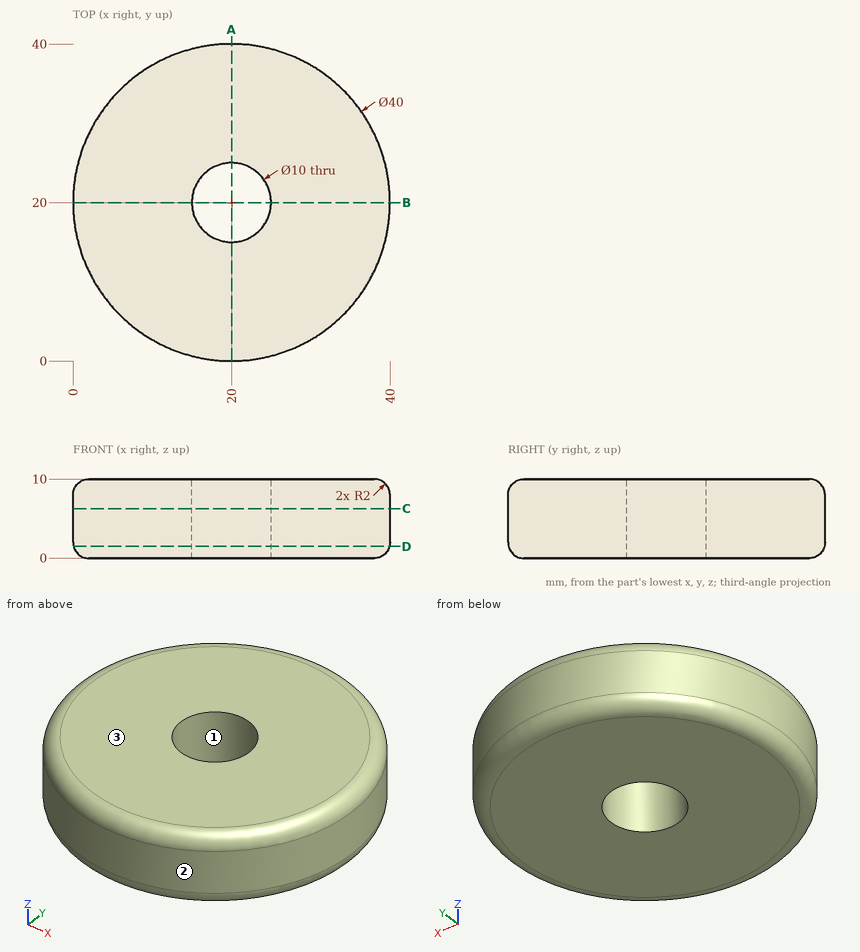
Geometry: see drawing. Coordinates: mm, zero at the bounding-box minimum. Round coordinates to 2 decimals unless told otherwise and drop trailing zeros. Loops run counter-clockwise (first coordinate to the right, second up) from the corner with the lowest first, then second, coordinate; pieces in that order, holes last. Notation, with made-up numbers: (38.5, 11.5) - (50.5, 11.5) arc R18 cw to (50.5, 32.5) - close; hole circle Ø5 at (29.25, -25). An arc over 180 degrees is marked (long way). Use CSV: the item, a comma, the result in double quotes.
Q1. Ray query, line 1 along Y through (x, z) = (20, 4); line 2 along Y through (x, z) = (17, 8); line 3 along Y through (x, z) = (36.5, 2.75). Return the intervals inside material, ascending.
Reported:
line 1,"0 to 15, 25 to 40"
line 2,"0.23 to 16, 24 to 39.77"
line 3,"8.7 to 31.3"
Q2. Section query C-C, the plane z = 6.25. Output: boundary loops of the cut face in (x, y), then the cut area to 3 significant figures.
Reported:
outline,"circle Ø40 at (20, 20); hole circle Ø10 at (20, 20)"
area,"1,180 mm^2"
Q3. Mould query, pull axis Y, two halves, no side actions, for the marked faces 1, 2 and 3. Classes: pulls with the +Y half, pulls with the -Y half, needs draft (parallel to the pull), parting line crosses it, or undercut.
Reported:
face 1,"undercut"
face 2,"parting line crosses it"
face 3,"needs draft"
Q4. Section query A-A, the plane x = 20. Output: boundary loops of the cut face in (y, z).
Reported:
outline,"(0, 2) arc R2 ccw to (2, 0) - (15, 0) - (15, 10) - (2, 10) arc R2 ccw to (0, 8) - close; (25, 0) - (38, 0) arc R2 ccw to (40, 2) - (40, 8) arc R2 ccw to (38, 10) - (25, 10) - close"
Q5. Pin query (flat end, axial travel): pin 1 Ø1.5 at (x, z) = (30, 3) entering from -Y; pin 2 Ø3 at (y, z) = (15, 8.5) entering from +X; pin 3 Ø1.5 at (x, z) = (5, 7.5) entering from -Y; pin 4 Ø9 at (x, y) = (20, 20) entering from -Z. Return the tip coordinate at first contact, or that it passes through.
Reported:
pin 1,"y = 2.27"
pin 2,"x = 39.68"
pin 3,"y = 5.97"
pin 4,"through"
Q6. Section query D-D, the plane z = 1.5. Output: boundary loops of the cut face in (x, y), then the cut area to 3 significant figures.
Reported:
outline,"circle Ø39.87 at (20, 20); hole circle Ø10 at (20, 20)"
area,"1,170 mm^2"
